Model file for the job. Use its own axes, mm. Coordinates: 2 decimals unless noted, no trailing zeros. Order: outer loops, then holes, each group sorted by start corner. A loop starts at its lowest first (then second) coordinate and runs counter-clockwise, first axis right, second up. Notation, with made-up numbers: (11, 82) - (17, 82) arc R21 ccw to (17, 89) - close; hole circle Ø10 at (-14, 48). An arc over 180 degrees is marked (long way). Put each result on its own line as item: value. Start each with the question number.
```python
from build123d import *

# Parameters (mm, degrees)
F1_DEPTH      = 147.193
F1_DEPTH_BACK = 147.193
F3_DEPTH      = 186.182


# Not quite as in the source:
# - a length typed as a fraction of an inch, garbled in the dataset ("3 / 203.2 mm" for 3/8 in), is restored


with BuildPart() as f1:
    # F0 (on Right) → F1 (new body, two sides)
    with BuildSketch(Plane.YZ) as f1_sk:
        with BuildLine():
            ThreePointArc((-155.7030739649, 130.5633668295), (-55.3860759172, 92.0728226971), (0, 0))
            Line((0, 0), (2.794, 0))
            ThreePointArc((2.794, 0), (-53.8777768496, 93.5114749264), (-155.7030739649, 133.3573668295))
            Line((-155.7030739649, 133.3573668295), (-155.7030739649, 130.5633668295))
        make_face()
    extrude(amount=-F1_DEPTH)
    extrude(f1_sk.sketch, amount=F1_DEPTH_BACK)

    # F2 (on Top) → F3 (cut)
    with BuildSketch(Plane.XY):
        with BuildLine():
            ThreePointArc((-128.6797374487, -155.7030739649), (-141.8112510122, -150.4712953815), (-147.193, -137.4005290135))
            Line((-147.193, -137.4005290135), (-161.3427400589, -137.4005290135))
            Line((-161.3427400589, -137.4005290135), (-161.3427400589, -161.3346251115))
            Line((-161.3427400589, -161.3346251115), (-129.2428970337, -161.3346251115))
            Line((-129.2428970337, -161.3346251115), (-128.6797374487, -155.7030739649))
        make_face()
        with BuildLine():
            Line((128.6797374487, -155.7030739649), (129.2428970337, -161.3346251115))
            Line((129.2428970337, -161.3346251115), (161.3427400589, -161.3346251115))
            Line((161.3427400589, -161.3346251115), (161.3427400589, -137.4005290135))
            Line((161.3427400589, -137.4005290135), (147.193, -137.4005290135))
            ThreePointArc((147.193, -137.4005290135), (141.8112510122, -150.4712953815), (128.6797374487, -155.7030739649))
        make_face()
    extrude(amount=F3_DEPTH, mode=Mode.SUBTRACT)


solid = f1.part
```
Item 1: Slice it at B-B, the plane y = -111. Give the cut face in (x, z), plus the area to 3 significant figures.
Item 2: Wall check: line 1 along Y through (x, z) = (90, 116.5); line 2 along Z through (x, y) = (113, -133.5); line 3 along Y through (x, z) = (-83.5, 54). Give the ranges that are in metal, low to high.
Item 3: Slice it at A-A, the plane x = -12. Give the cut face in (y, z).
Item 4: Flat gauge pins, fed straight in: pin 1 Ø5 at (x, y) = (6.5, -102.5) entering from +Z; pin 2 Ø1 at (x, y) = (-22, -17.5) entering from -Z; pin 3 Ø5 at (x, z) = (-0.5, 83) entering from +Y. Where does each tip first touch, or does it go through?
Here are the results:
1. outline: (-147.19, 122.76) - (147.19, 122.76) - (147.19, 125.21) - (-147.19, 125.21) - close
1. area: 722 mm^2
2. line 1: y = -94.56 to -89.33
2. line 2: z = 128.28 to 130.86
2. line 3: y = -22.05 to -19.43
3. outline: (-155.7, 130.56) arc R165.1 cw to (0, 0) - (2.79, 0) arc R170.47 ccw to (-155.7, 133.36) - close
4. pin 1: stops at z = 123.14
4. pin 2: stops at z = 45.48
4. pin 3: stops at y = -40.06
